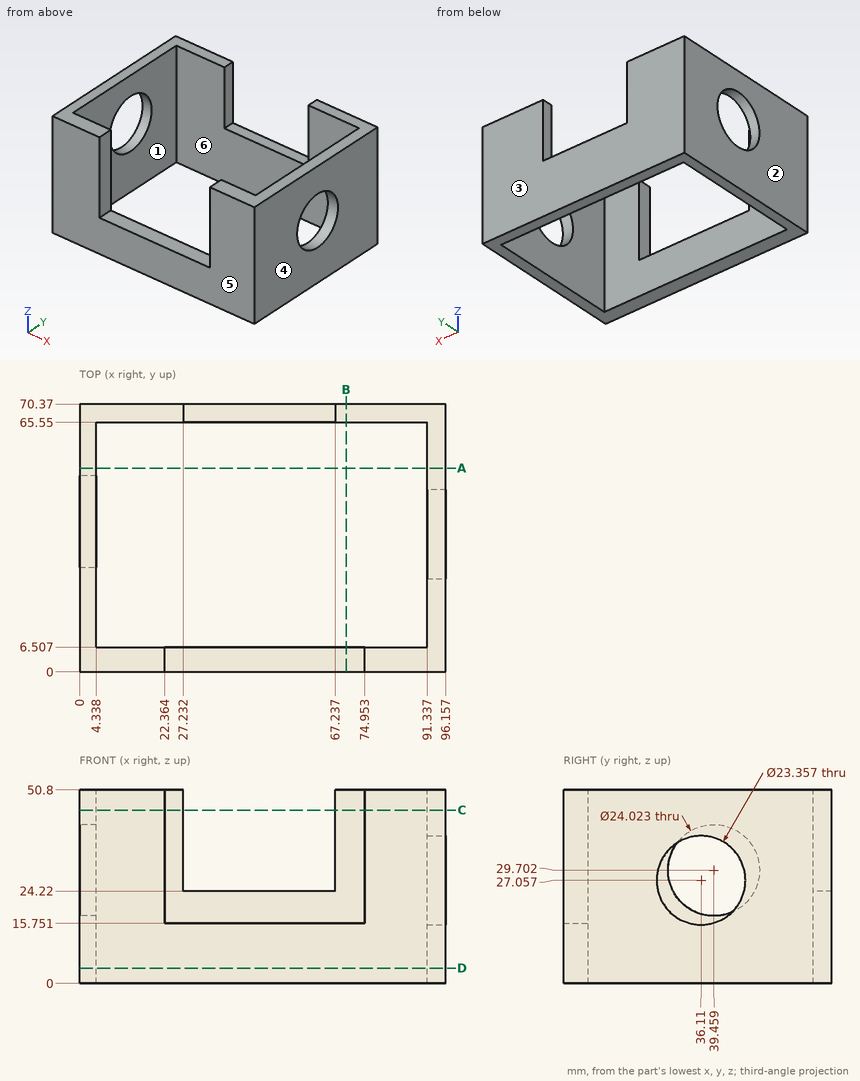
For this review, use the dimensioned drawing (mm, ordinates from the lowest corner) and the shaded views. A direction names the side the tool comes from. Give positions to 0.01 mm unless a question says otherwise; leave off trailing zeros. Loops run counter-clockwise (first coordinate to the right, second up) from the corner with the lowest first, then second, coordinate; pieces in that order, holes last. Notation, with made-up numbers: (62.5, -6) -> (108.5, -6) arc R10 cw to (108.5, 1) -> close; hole circle Ø8 at (-28, 62.5). An arc over 180 degrees is marked (long way). Use CSV: the item, a comma, the result in double quotes.
1. Consider section D-D, the plane z = 4. Write out the cut boundary in (x, y).
Result:
outline,"(0, 0) -> (96.16, 0) -> (96.16, 70.37) -> (0, 70.37) -> close; hole (4.34, 6.51) -> (91.34, 6.51) -> (91.34, 65.55) -> (4.34, 65.55) -> close"
2. For P1, Ø5.5, axis at x = 53.5, y = 68.5, coming from the +Z side; P2, Ø3.5, axis at x = 55, y = 3, coming from the +Z side, all flat-tipped, find the tip position at first contact; note any pin that passes through.
Result:
P1,"stops at z = 24.22"
P2,"stops at z = 15.75"
3. Consider section A-A, the plane y = 53.5. Write out the cut boundary in (x, z), then the cut area to 3 significant figures.
Result:
outline,"(0, 0) -> (4.34, 0) -> (4.34, 50.8) -> (0, 50.8) -> close; (91.34, 0) -> (96.16, 0) -> (96.16, 50.8) -> (91.34, 50.8) -> close"
area,"465 mm²"
4. The part is to be moulded in two halves that separate along X. For the marked faces 1, 2, 3 and 4, say which applies: +X half, -X half, draft (parallel to the pull), parting line (faces both ways), or undercut.
Result:
face 1,"undercut"
face 2,"-X half"
face 3,"draft"
face 4,"+X half"
5. Consider section C-C, the plane z = 45.5. Write out the cut boundary in (x, y).
Result:
outline,"(0, 0) -> (22.36, 0) -> (22.36, 6.51) -> (4.34, 6.51) -> (4.34, 65.55) -> (27.23, 65.55) -> (27.23, 70.37) -> (0, 70.37) -> close; (67.24, 65.55) -> (91.34, 65.55) -> (91.34, 6.51) -> (74.95, 6.51) -> (74.95, 0) -> (96.16, 0) -> (96.16, 70.37) -> (67.24, 70.37) -> close"
6. Consider section B-B, the plane x = 70. Write out the cut boundary in (y, z).
Result:
outline,"(0, 0) -> (6.51, 0) -> (6.51, 15.75) -> (0, 15.75) -> close; (65.55, 0) -> (70.37, 0) -> (70.37, 50.8) -> (65.55, 50.8) -> close"
7. Machinability: for the marked faces 5 and 6, which of the approach directions +Z, -Z, +X, -X, +Y, -Y give a long, thin tool a straight path to every point of the face, cutting with its end or side? Answer none if there is none.
Result:
face 5,"+Z, -Z, +X, -X, -Y"
face 6,"+Z, -Z"
8. To check wall thickness, follow probe 1 along X at (y, z) = (12.5, 7); probe 2 along Y at (x, z) = (73, 14); probe 3 along X at (y, z) = (5.5, 23). State the ranges of each line that lie inside material, in increasing order. Write a range as from..to.
Result:
probe 1,"x = 0..4.34, 91.34..96.16"
probe 2,"y = 0..6.51, 65.55..70.37"
probe 3,"x = 0..22.36, 74.95..96.16"
